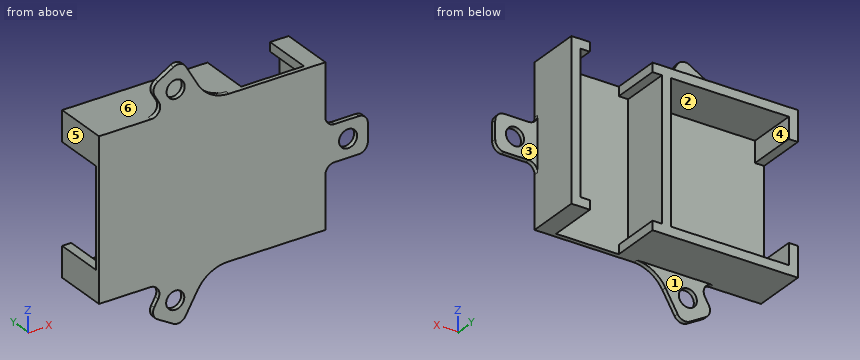
```python
from build123d import *

# Parameters (mm, degrees)
BOSS_EXTRUDE1_DEPTH   = 11
BOSS_EXTRUDE1_2_DEPTH = 11
SKETCH2_R             = 2
BOSS_EXTRUDE2_DEPTH   = 1


with BuildPart() as part:
    # Sketch1 → Boss-Extrude1 (new body)
    with BuildSketch(Plane(origin=(0, 0, 0), x_dir=(1, 0, 0), z_dir=(0, 1, 0))):
        Polygon((-26.926443894, -15.5), (-0.926443894, -15.5), (-0.926443894, 15.5), (-26.926443894, 15.5), (-26.926443894, 10.846689955), (-28.926443894, 10.846689955), (-28.926443894, 17.5), (3.157388066, 17.5), (3.157388066, 15.5), (1.073556106, 15.5), (1.073556106, -15.5), (3.157388066, -15.5), (3.157388066, -17.5), (-28.926443894, -17.5), (-28.926443894, -10.846689955), (-26.926443894, -10.846689955), align=None)
    extrude(amount=BOSS_EXTRUDE1_DEPTH)



with BuildPart() as body_2:
    # Sketch1 → Boss-Extrude1 2 (new body)
    with BuildSketch(Plane(origin=(0, 0, 0), x_dir=(1, 0, 0), z_dir=(0, 1, 0))):
        Polygon((19.073556106, 15.5), (19.073556106, -15.5), (16.989724146, -15.5), (16.989724146, -17.5), (21.073556106, -17.5), (21.073556106, 17.5), (16.989724146, 17.5), (16.989724146, 15.5), align=None)
    extrude(amount=BOSS_EXTRUDE1_2_DEPTH)


with BuildPart() as part_1:
    add(part.part)

    add(body_2.part)  # Boss-Extrude2 merges body 2
    # Sketch2 → Boss-Extrude2 (add)
    with BuildSketch(Plane.XZ):
        with BuildLine():
            Line((-28.926443894, 17.5), (-17.408269171, 17.5))
            ThreePointArc((-17.408269171, 17.5), (-15.676218364, 18.5), (-15.676218364, 20.5))
            Line((-15.676218364, 20.5), (-16.624724435, 22.142860706))
            ThreePointArc((-16.624724435, 22.142860706), (-16.82452528, 23.660498796), (-15.892673627, 24.874911513))
            Line((-15.892673627, 24.874911513), (-12.469020781, 26.851558406))
            ThreePointArc((-12.469020781, 26.851558406), (-10.951382691, 27.051359251), (-9.736969974, 26.119507598))
            Line((-9.736969974, 26.119507598), (-7.056413095, 21.476646892))
            ThreePointArc((-7.056413095, 21.476646892), (-4.145305527, 18.565539323), (-0.168658635, 17.5))
            Line((-0.168658635, 17.5), (21.073556106, 17.5))
            Line((21.073556106, 17.5), (21.073556106, 5.976646892))
            ThreePointArc((21.073556106, 5.976646892), (21.659342544, 4.56243333), (23.073556106, 3.976646892))
            Line((23.073556106, 3.976646892), (28.434669863, 3.976646892))
            ThreePointArc((28.434669863, 3.976646892), (29.848883425, 3.390860454), (30.434669863, 1.976646892))
            Line((30.434669863, 1.976646892), (30.434669863, -1.976646892))
            ThreePointArc((30.434669863, -1.976646892), (29.848883425, -3.390860454), (28.434669863, -3.976646892))
            Line((28.434669863, -3.976646892), (23.073556106, -3.976646892))
            ThreePointArc((23.073556106, -3.976646892), (21.659342544, -4.56243333), (21.073556106, -5.976646892))
            Line((21.073556106, -5.976646892), (21.073556106, -17.5))
            Line((21.073556106, -17.5), (-0.864905973, -17.5))
            ThreePointArc((-0.864905973, -17.5), (-4.494457946, -18.60652774), (-7.146873061, -21.319965636))
            Line((-7.146873061, -21.319965636), (-9.827429939, -25.962826342))
            ThreePointArc((-9.827429939, -25.962826342), (-11.041842657, -26.894677994), (-12.559480747, -26.694877149))
            Line((-12.559480747, -26.694877149), (-15.983133593, -24.718230257))
            ThreePointArc((-15.983133593, -24.718230257), (-16.914985245, -23.50381754), (-16.7151844, -21.98617945))
            Line((-16.7151844, -21.98617945), (-15.857138295, -20.5))
            ThreePointArc((-15.857138295, -20.5), (-15.857138295, -18.5), (-17.589189102, -17.5))
            Line((-17.589189102, -17.5), (-28.926443894, -17.5))
            Line((-28.926443894, -17.5), (-28.926443894, 17.5))
        make_face()
        with Locations(Location((26.073556106, 0, 0), (0, 0, 270))):
            Circle(SKETCH2_R, mode=Mode.SUBTRACT)
        with Locations(Location((-12.090750291, -21.929718401, 0), (0, 0, 270))):
            Circle(SKETCH2_R, mode=Mode.SUBTRACT)
        with Locations(Location((-12.000290326, 22.086399657, 0), (0, 0, 270))):
            Circle(SKETCH2_R, mode=Mode.SUBTRACT)
    extrude(amount=BOSS_EXTRUDE2_DEPTH)


solid = part_1.part
```
The model under review builds one solid part; all positions refer to its coordinate system, in mm. Face numbers are marked on the shaded views. A direction names the side the tool comes from. Coordinates: 2 decimals unless noted, no trailing zeros. Write each loop counter-clockwise with the first axis right and the second up, starting at its lowest first coordinate (ties: lowest second). Pieces come first, ordered by that corner, then holes.
1) We need section B-B on y = 3.5. State the section outline as (x, z) points.
2) Machinability: for the marked faces 1, 2 and 3, which of the approach directions +Z, -Z, +X, -X, +Y, -Y give a long, thin tool a straight path to every point of the face, cutting with its end or side? Answer none if there is none.
3) We need section A-A on z = 0. State the section outline as (x, y) points.
4) Clearance check with flat-ended pins moving along their axes: pin 1 Ø1 at (y, z) = (6, 16.5) entering from +X; pin 2 Ø0.6 at (x, y) = (-28, 4) entering from +Z; pin 3 Ø1.7 at (x, y) = (2, 3) entering from -Z; pin 4 Ø5 at (x, y) = (24, 7.5) entering from +Z. State where each tip first meets the part, or that it passes through.
5) We need section D-D on z = 23. State the section outline as (x, y) points.
6) To check wall thickness, follow probe 1 along X at (y, z) = (5, 11); probe 2 along X at (y, z) = (8.5, 17); probe 3 along Z at (x, y) = (-24, 5). State the ranges of each line that lie inside material, in increasing order.
7) The part is to be moulded in two halves that separate along Z. For the marked faces 4, 5 and 6, say which applies: pulls with the +Z half, pulls with the -Z half, needs draft (parallel to the pull), parting line crosses it, or undercut.
8) We need section C-C on x = 4. State the section outline as (y, z) points, then the cut area to 3 significant figures.
Answer list:
1. outline: (-28.93, -17.5) - (3.16, -17.5) - (3.16, -15.5) - (1.07, -15.5) - (1.07, 15.5) - (3.16, 15.5) - (3.16, 17.5) - (-28.93, 17.5) - (-28.93, 10.85) - (-26.93, 10.85) - (-26.93, 15.5) - (-0.93, 15.5) - (-0.93, -15.5) - (-26.93, -15.5) - (-26.93, -10.85) - (-28.93, -10.85) - close; (16.99, -17.5) - (21.07, -17.5) - (21.07, 17.5) - (16.99, 17.5) - (16.99, 15.5) - (19.07, 15.5) - (19.07, -15.5) - (16.99, -15.5) - close
2. face 1: -Z, +X, -X, +Y
2. face 2: +Y
2. face 3: +Z, -Z, +X, +Y
3. outline: (-28.93, -1) - (24.07, -1) - (24.07, 0) - (21.07, 0) - (21.07, 11) - (19.07, 11) - (19.07, 0) - (1.07, 0) - (1.07, 11) - (-0.93, 11) - (-0.93, 0) - (-28.93, 0) - close; (28.07, -1) - (30.43, -1) - (30.43, 0) - (28.07, 0) - close
4. pin 1: stops at x = 21.07
4. pin 2: stops at z = 17.5
4. pin 3: stops at z = -17.5
4. pin 4: passes through
5. outline: (-16.89, -1) - (-13.78, -1) - (-13.78, 0) - (-16.89, 0) - close; (-10.22, -1) - (-7.94, -1) - (-7.94, 0) - (-10.22, 0) - close
6. probe 1: x = -28.93 to -26.93, -0.93 to 1.07, 19.07 to 21.07
6. probe 2: x = -28.93 to 3.16, 16.99 to 21.07
6. probe 3: z = -17.5 to -15.5, 15.5 to 17.5
7. face 4: undercut
7. face 5: needs draft
7. face 6: pulls with the +Z half
8. outline: (-1, -17.5) - (0, -17.5) - (0, 17.5) - (-1, 17.5) - close
8. area: 35.0 mm2
